The model under review builds one solid part; all positions refer to its coordinate system, in mm. Face numbers are marked on the shaded views. A direction names the side the tool comes from. Give positions to 0.01 mm unless a question says otherwise; leave off trailing zeros. Loops run counter-clockwise (first coordinate to the right, second up) from the corner with the lowest first, then second, coordinate; pieces in that order, holes last. Notation, with made-up numbers: (68.5, 3.5) - (99.5, 3.5) arc R10 ccw to (99.5, 15.5) - close; hole circle Ø1 at (23.25, -28.5). An arc over 180 degrees is marked (long way). Return JSON: item names as keys, results as strings. Group by question number.
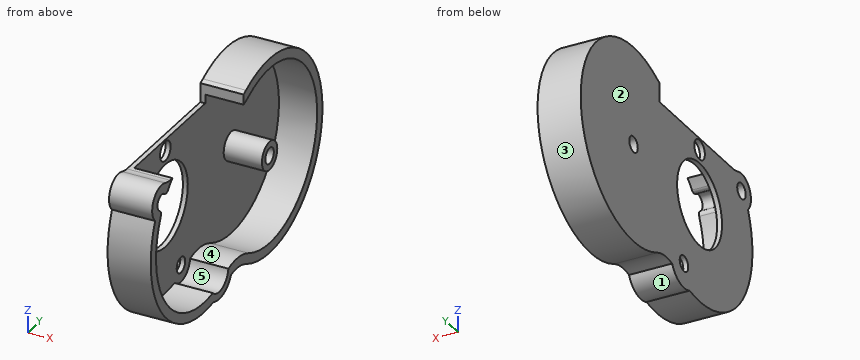
```python
from build123d import *

# Parameters (mm, degrees)
BOSS_EXTRUDE1_DEPTH = 8.8
SKETCH1_3_R         = 1.9950000000003372
SKETCH1_3_R_2       = 8.499000000001052
SKETCH1_3_R_3       = 1.5999999999998604
SKETCH1_3_R_4       = 2.9000000000004036
BOSS_EXTRUDE2_DEPTH = 1
SKETCH1_4_R         = 2.9000000000004036
SKETCH1_4_R_2       = 1.5999999999998604
BOSS_EXTRUDE3_DEPTH = 8.8
FILLET1_R           = 1


with BuildPart() as part:
    # Sketch1 → Boss-Extrude1 (new body)
    with BuildSketch(Plane(origin=(-9277.020495484805, 0, 0), x_dir=(0, 0, -1), z_dir=(1, 0, 0))):
        with BuildLine():
            Line((-5181.361026538003, -2712.2298566105233), (-5181.361026538003, -2713.1295442369124))
            ThreePointArc((-5181.361026538003, -2713.1295442369124), (-5181.449009948379, -2714.0634034464592), (-5181.7098637473055, -2714.9643970087795))
            ThreePointArc((-5181.7098637473055, -2714.9643970087795), (-5180.298716040606, -2719.319524523044), (-5175.754002429446, -2718.7681156836497))
            ThreePointArc((-5175.754002429446, -2718.7681156836493), (-5155.268489112517, -2716.0470361610683), (-5148.125988175469, -2696.6551510028244))
            ThreePointArc((-5148.125988175468, -2696.6551510028244), (-5147.923825496746, -2692.8741534881237), (-5150.429715151682, -2690.0356100249855))
            ThreePointArc((-5150.429715151682, -2690.0356100249855), (-5150.672402006578, -2687.1467824336814), (-5149.869641086049, -2684.3611412747578))
            ThreePointArc((-5149.869641086049, -2684.3611412747578), (-5167.766026538003, -2655.432569846187), (-5185.662411989956, -2684.361141274758))
            ThreePointArc((-5185.662411989956, -2684.361141274758), (-5185.445898231984, -2684.832832292979), (-5185.260425515467, -2685.3175698461864))
            Line((-5185.2604255154665, -2685.3175698461864), (-5183.1689314111645, -2685.3175698461864))
            ThreePointArc((-5183.1689314111645, -2685.3175698461864), (-5183.475000193814, -2684.375475532257), (-5183.87277344476, -2683.4682841319004))
            ThreePointArc((-5183.872773444761, -2683.468284131901), (-5167.766026538003, -2657.432569846187), (-5151.659279631244, -2683.4682841319004))
            ThreePointArc((-5151.659279631244, -2683.4682841319004), (-5152.684326847257, -2687.2014849950892), (-5152.214633681771, -2691.0442572769534))
            ThreePointArc((-5152.214633681771, -2691.044257276954), (-5149.350375503743, -2693.339145363929), (-5150.110119114768, -2696.929866167285))
            ThreePointArc((-5150.110119114768, -2696.929866167285), (-5157.293990334202, -2715.0728040569593), (-5176.7849023498975, -2716.0101139109493))
            ThreePointArc((-5176.7849023498975, -2716.0101139109493), (-5179.250079105888, -2717.6157486981815), (-5178.709438757866, -2714.723886405067))
            ThreePointArc((-5178.709438757866, -2714.723886405067), (-5180.098441740306, -2713.544073775103), (-5181.361026538003, -2712.2298566105233))
        make_face()
    extrude(amount=BOSS_EXTRUDE1_DEPTH)

    # Sketch1<3> → Boss-Extrude2 (add)
    with BuildSketch(Plane(origin=(-9277.020495484805, 0, 0), x_dir=(0, 0, -1), z_dir=(1, 0, 0))):
        with BuildLine():
            Line((-5181.361026538003, -2685.3175698461864), (-5181.361026538003, -2712.2298566105233))
            ThreePointArc((-5181.361026538003, -2712.2298566105233), (-5180.098441740306, -2713.544073775103), (-5178.709438757866, -2714.723886405067))
            ThreePointArc((-5178.709438757866, -2714.723886405067), (-5177.471973970118, -2714.9552333108672), (-5176.7849023498975, -2716.0101139109493))
            ThreePointArc((-5176.7849023498975, -2716.0101139109493), (-5175.822472884072, -2716.5289567784425), (-5174.830317408971, -2716.98840852897))
            ThreePointArc((-5174.830317408971, -2716.98840852897), (-5156.424427633244, -2714.409984996477), (-5150.110119114768, -2696.929866167285))
            ThreePointArc((-5150.110119114768, -2696.929866167285), (-5149.350375503743, -2693.339145363929), (-5152.214633681771, -2691.044257276954))
            ThreePointArc((-5152.214633681771, -2691.0442572769534), (-5152.429634860403, -2690.2883766387154), (-5152.584616128909, -2689.5179469842446))
            ThreePointArc((-5152.584616128909, -2689.5179469842446), (-5152.596121525538, -2686.4205875195544), (-5151.659279631244, -2683.4682841319004))
            ThreePointArc((-5151.659279631244, -2683.4682841319004), (-5167.766026538003, -2657.432569846187), (-5183.872773444761, -2683.468284131901))
            ThreePointArc((-5183.87277344476, -2683.4682841319004), (-5183.475000193814, -2684.375475532257), (-5183.1689314111645, -2685.3175698461864))
            Line((-5183.1689314111645, -2685.3175698461864), (-5181.361026538003, -2685.3175698461864))
        make_face()
        with Locations(Location((-5179.016026538003, -2700.4325698461867, 0), (0, 0, 180))):
            Circle(SKETCH1_3_R, mode=Mode.SUBTRACT)
        with Locations(Location((-5167.766026538003, -2700.432569846186, 0), (0, 0, 180))):
            Circle(SKETCH1_3_R_2, mode=Mode.SUBTRACT)
        with Locations(Location((-5152.646026538003, -2694.5175698461867, 0), (0, 0, 180))):
            Circle(SKETCH1_3_R_3, mode=Mode.SUBTRACT)
        with Locations(Location((-5167.766026538003, -2675.4325698461867, 0), (0, 0, 180))):
            Circle(SKETCH1_3_R_4, mode=Mode.SUBTRACT)
    extrude(amount=BOSS_EXTRUDE2_DEPTH)

    # Sketch1<4> → Boss-Extrude3 (add)
    with BuildSketch(Plane(origin=(-9277.020495484805, 0, 0), x_dir=(0, 0, -1), z_dir=(1, 0, 0))):
        with Locations(Location((-5167.766026538003, -2675.4325698461867, 0), (0, 0, 180))):
            Circle(SKETCH1_4_R)
        with Locations((-5167.766026538003, -2675.4325698461867)):
            Circle(SKETCH1_4_R_2, mode=Mode.SUBTRACT)
    extrude(amount=BOSS_EXTRUDE3_DEPTH)

    # Fillet1
    fillet1_edges = [part.edges().sort_by_distance(p)[0] for p in [
        (-9272.120495484805, -2716.0101139109493, 5176.7849023498975),
        (-9272.120495484805, -2714.723886405067, 5178.709438757866),
    ]]
    fillet(fillet1_edges, radius=FILLET1_R)


solid = part.part
```
1) We need section D-D, the plane z = 5172. Write out the cut boundary in (x, y), plus the area to 3 significant figures.
2) We need section C-C, the plane x = -9272. Count the separate pieces of the cut face and the enclosed holes in it, plus the area to 3 significant figures.
3) For pin 1 Ø2 at (y, z) = (-2711, 5172) entering from +X; pin 2 Ø4.5 at (x, z) = (-9270.5, 5183) entering from -Y; pin 3 Ø2.5 at (y, z) = (-2675.43, 5167.77) entering from -X; pin 4 Ø3 at (x, y) = (-9274, -2676) entering from +Z, all flat-tipped, find the tip position at first contact; note any pin that passes through.
4) We need section A-A, the plane z = 5164. Write out the cut boundary in (x, y), plus the area to 3 significant figures.
5) Draft analysis for pull direction Y (two halves, no side actions). For the marked faces 1 and 2, state which applies: +Y half, -Y half, draft (parallel to the pull), parting line (faces both ways), or undercut.
6) Tool access review of the marked faces 3, 4 and 5: name each direction out of +Z, -Z, +X, -X, +Y, -Y from which nothing blocks a thin tool from reaching the whole face with its end or side.
7) To check wall thickness, follow line 1 (Y direction, x = -9274, z = 5162); line 2 (X direction, y = -2696.5, z = 5176.5); line 3 (Y direction, x = -9269.25, z = 5173). State the ranges of each line that lie inside material, in increasing order.
8) We need section B-B, the plane y = -2663.5. Write out the cut boundary in (x, z).
Findings:
{
 "1": {"outline": "(-9277.02, -2719.98) - (-9268.22, -2719.98) - (-9268.22, -2717.93) - (-9276.02, -2717.93) - (-9276.02, -2707.8) - (-9277.02, -2707.8) - close; (-9277.02, -2693.06) - (-9276.02, -2693.06) - (-9276.02, -2657.94) - (-9268.22, -2657.94) - (-9268.22, -2655.89) - (-9277.02, -2655.89) - close", "area": "81.4 mm^2"},
 "2": {"separate pieces": "2", "enclosed holes": "1", "area": "305 mm^2"},
 "3": {"pin 1": "stops at x = -9276.02", "pin 2": "stops at y = -2718.98", "pin 3": "passes through", "pin 4": "stops at z = 5187.77"},
 "4": {"outline": "(-9277.02, -2720.07) - (-9268.22, -2720.07) - (-9268.22, -2718.03) - (-9276.02, -2718.03) - (-9276.02, -2708.05) - (-9277.02, -2708.05) - close; (-9277.02, -2692.81) - (-9276.02, -2692.81) - (-9276.02, -2657.83) - (-9268.22, -2657.83) - (-9268.22, -2655.79) - (-9277.02, -2655.79) - close", "area": "80.9 mm^2"},
 "5": {"face 1": "undercut", "face 2": "draft"},
 "6": {"face 3": "+X, -X", "face 4": "+X", "face 5": "+Z, +X"},
 "7": {"line 1": "y = -2719.58 to -2717.48, -2658.38 to -2656.28", "line 2": "x = -9277.02 to -9276.02", "line 3": "y = -2719.74 to -2717.65, -2658.21 to -2656.13"},
 "8": {"outline": "(-9277.02, 5151.72) - (-9268.22, 5151.72) - (-9268.22, 5154.29) - (-9276.02, 5154.29) - (-9276.02, 5181.24) - (-9268.22, 5181.24) - (-9268.22, 5183.82) - (-9277.02, 5183.82) - close"}
}
